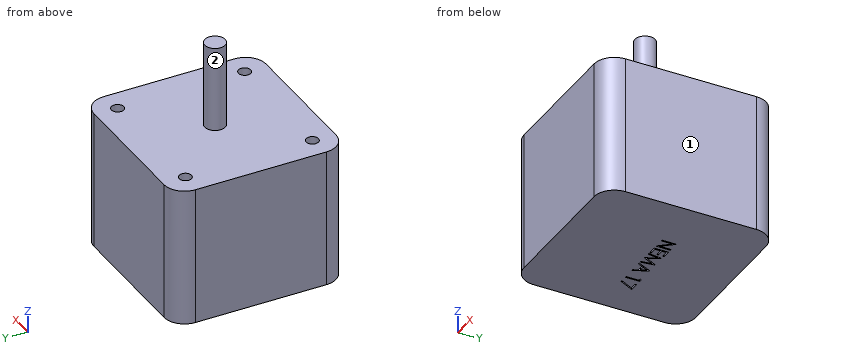
```python
from build123d import *

# Parameters (mm, degrees)
SZKIC1_W                    = 42
SZKIC1_H                    = 42
DODANIE_WYCI_GNI_CIE1_DEPTH = 34
SZKIC2_R                    = 1.5
WYTNIJ_WYCI_GNI_CIE1_DEPTH  = 11
SZKIC6_R                    = 1.5
WYTNIJ_WYCI_GNI_CIE2_DEPTH  = 11
SZKIC7_R                    = 1.5
WYTNIJ_WYCI_GNI_CIE3_DEPTH  = 11
SZKIC8_R                    = 1.5
WYTNIJ_WYCI_GNI_CIE4_DEPTH  = 11
ZAOKR_GLENIE1_R             = 5
SZKIC9_R                    = 2.5
DODANIE_WYCI_GNI_CIE4_DEPTH = 21
WYTNIJ_WYCI_GNI_CIE5_DEPTH  = 1


with BuildPart() as part:
    # Szkic1 → Dodanie-wyciągnięcie1 (new body)
    with BuildSketch(Plane.XY):
        Rectangle(SZKIC1_W, SZKIC1_H)
    extrude(amount=DODANIE_WYCI_GNI_CIE1_DEPTH)

    # Szkic2 → Wytnij-wyciągnięcie1 (cut)
    with BuildSketch(Plane.XY.offset(34)):
        with Locations((15.5, 15.5)):
            Circle(SZKIC2_R)
    extrude(amount=-WYTNIJ_WYCI_GNI_CIE1_DEPTH, mode=Mode.SUBTRACT)

    # Szkic6 → Wytnij-wyciągnięcie2 (cut)
    with BuildSketch(Plane.XY.offset(34)):
        with Locations((-15.5, 15.5)):
            Circle(SZKIC6_R)
    extrude(amount=-WYTNIJ_WYCI_GNI_CIE2_DEPTH, mode=Mode.SUBTRACT)

    # Szkic7 → Wytnij-wyciągnięcie3 (cut)
    with BuildSketch(Plane.XY.offset(34)):
        with Locations((-15.5, -15.5)):
            Circle(SZKIC7_R)
    extrude(amount=-WYTNIJ_WYCI_GNI_CIE3_DEPTH, mode=Mode.SUBTRACT)

    # Szkic8 → Wytnij-wyciągnięcie4 (cut)
    with BuildSketch(Plane.XY.offset(34)):
        with Locations((15.5, -15.5)):
            Circle(SZKIC8_R)
    extrude(amount=-WYTNIJ_WYCI_GNI_CIE4_DEPTH, mode=Mode.SUBTRACT)

    # Zaokrąglenie1
    zaokr_glenie1_edges = [part.edges().sort_by_distance(p)[0] for p in [
        (21, -21, 17),
        (-21, -21, 17),
        (-21, 21, 17),
        (21, 21, 17),
    ]]
    fillet(zaokr_glenie1_edges, radius=ZAOKR_GLENIE1_R)

    # Szkic9 → Dodanie-wyciągnięcie4 (add)
    with BuildSketch(Plane.XY.offset(34)):
        with Locations(Location((0, 0, 0), (0, 0, 180))):
            Circle(SZKIC9_R)
    extrude(amount=DODANIE_WYCI_GNI_CIE4_DEPTH)

    # Szkic11 → Wytnij-wyciągnięcie5 (cut)
    # profile 1 of 6: a face of its own
    with BuildSketch(Plane(origin=(0, 0, 0), x_dir=(-1, 0, 0), z_dir=(0, 0, -1))):
        Polygon((-7.658605606, 0.036910524), (-7.658605606, 3.536910524), (-7.592700157, 3.536910524), (-5.280400478, 0.782202992), (-5.280400478, 3.536910524), (-4.966297913, 3.536910524), (-4.966297913, 0.036910524), (-5.037812336, 0.036910524), (-7.344503042, 2.78530796), (-7.344503042, 0.036910524), align=None)
    # profile 2 of 6: a face of its own
    with BuildSketch(Plane(origin=(0, 0, 0), x_dir=(-1, 0, 0), z_dir=(0, 0, -1))):
        Polygon((-4.068862016, 3.536910524), (-2.094503042, 3.536910524), (-2.094503042, 3.177936165), (-3.754759452, 3.177936165), (-3.754759452, 2.101013088), (-2.094503042, 2.101013088), (-2.094503042, 1.742038729), (-3.754759452, 1.742038729), (-3.754759452, 0.395884883), (-2.094503042, 0.395884883), (-2.094503042, 0.036910524), (-4.068862016, 0.036910524), align=None)
    # profile 3 of 6: a face of its own
    with BuildSketch(Plane(origin=(0, 0, 0), x_dir=(-1, 0, 0), z_dir=(0, 0, -1))):
        Polygon((-1.645785093, 0.036910524), (-1.18374583, 3.536910524), (-1.138874035, 3.536910524), (0.306137984, 0.665115652), (1.747644394, 3.536910524), (1.793217311, 3.536910524), (2.258061061, 0.036910524), (1.942556253, 0.036910524), (1.607420035, 2.555340011), (0.343998561, 0.036910524), (0.27318526, 0.036910524), (-0.995144067, 2.560948986), (-1.329579163, 0.036910524), align=None)
    # profile 4 of 6: a face of its own
    with BuildSketch(Plane(origin=(0, 0, 0), x_dir=(-1, 0, 0), z_dir=(0, 0, -1))):
        Polygon((4.411907215, 3.536910524), (6.02729183, 0.036910524), (5.685845516, 0.036910524), (5.168417631, 1.158705396), (3.58177901, 1.158705396), (3.049627567, 0.036910524), (2.70677901, 0.036910524), (4.36703542, 3.536910524), align=None)
        Polygon((4.385965708, 2.854719018), (3.752151606, 1.517679755), (5.002952888, 1.517679755), align=None, mode=Mode.SUBTRACT)
    # profile 5 of 6: a face of its own
    with BuildSketch(Plane(origin=(0, 0, 0), x_dir=(-1, 0, 0), z_dir=(0, 0, -1))):
        Polygon((8.431438465, 3.536910524), (9.078573881, 3.536910524), (9.078573881, 0.036910524), (8.764471317, 0.036910524), (8.764471317, 3.177936165), (8.226009779, 3.177936165), align=None)
    # profile 6 of 6: a face of its own
    with BuildSketch(Plane(origin=(0, 0, 0), x_dir=(-1, 0, 0), z_dir=(0, 0, -1))):
        Polygon((10.604214907, 3.536910524), (12.758061061, 3.536910524), (10.918317471, -0.052833066), (10.646983337, 0.096505877), (12.22661074, 3.177936165), (10.604214907, 3.177936165), align=None)
    extrude(amount=-WYTNIJ_WYCI_GNI_CIE5_DEPTH, mode=Mode.SUBTRACT)


solid = part.part
```
The model under review builds one solid part; all positions refer to its coordinate system, in mm. Face numbers are marked on the shaded views. A direction names the side the tool comes from. Round coordinates to 2 decimals unless told otherwise and drop trailing zeros. Loops run counter-clockwise (first coordinate to the right, second up) from the corner with the lowest first, then second, coordinate; pieces in that order, holes last.
Item 1: Clearance check with flat-ended pins moving along their axes: pin 1 Ø10 at (y, z) = (-1.5, 48) entering from +X; pin 2 Ø1.5 at (x, y) = (-15, -15) entering from +Z; pin 3 Ø12 at (y, z) = (-13.5, 44) entering from -X; pin 4 Ø10 at (y, z) = (7, 43) entering from +X. State where each tip first meets the part, or that it passes through.
Determined:
pin 1: stops at x = 2.5
pin 2: stops at z = 23
pin 3: passes through
pin 4: stops at x = 1.5
Item 2: Take a section at B-B (y = 11.5). Write out the cut boundary in (x, z).
Determined:
outline: (-21, 0) - (21, 0) - (21, 34) - (-21, 34) - close
Item 3: Take a section at A-A (x = 6.5). Write out the cut boundary in (y, z).
Determined:
outline: (-21, 0) - (1.78, 0) - (1.78, 1) - (2.24, 1) - (2.24, 0) - (21, 0) - (21, 34) - (-21, 34) - close
Item 4: For the marked faces 1 and 2, list the 3-axis set-ups (+Z, -Z, +X, -X, +Y, -Y) from which the entire face can be reached by the end or side of a thin tool; tool diameter is ignored.
Determined:
face 1: +Z, -Z, +X, +Y, -Y
face 2: +Z
Item 5: For line 1 (Y direction, x = 15.5, z = 29); line 2 (X direction, y = -15, z = 27), list the stretches that pass through material, from the lowest coordinate up.
Determined:
line 1: y = -21 to -17, -14 to 14, 17 to 21
line 2: x = -21 to -16.91, -14.09 to 14.09, 16.91 to 21
